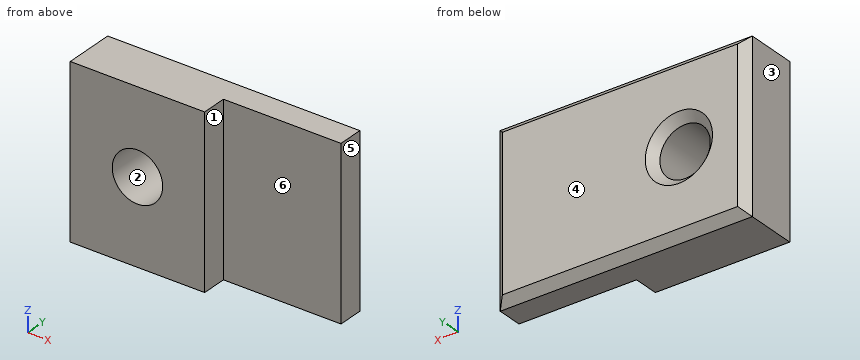
```python
from build123d import *

# Parameters (mm, degrees)
SKETCH1_W           = 30
SKETCH1_H           = 20
SKETCH1_R           = 3
BOSS_EXTRUDE1_DEPTH = 7
SKETCH2_OUTSIDE_W   = 39.346
SKETCH2_OUTSIDE_H   = 29.346
SKETCH2_OUTSIDE_W_2 = 16
SKETCH2_OUTSIDE_H_2 = 20
CUT_EXTRUDE1_DEPTH  = 3
CHAMFER1_SIZE       = 1


with BuildPart() as part:
    # Sketch1 → Boss-Extrude1 (new body)
    with BuildSketch(Plane(origin=(0, 0, 0), x_dir=(1, 0, 0), z_dir=(0, 1, 0))):
        with Locations((7, 0)):
            Rectangle(SKETCH1_W, SKETCH1_H)
        Circle(SKETCH1_R, mode=Mode.SUBTRACT)
    extrude(amount=BOSS_EXTRUDE1_DEPTH)

    # Sketch2 outside → Cut-Extrude1 (cut)
    with BuildSketch(Plane.XZ):
        with Locations((7, 0)):
            Rectangle(SKETCH2_OUTSIDE_W, SKETCH2_OUTSIDE_H)
        Rectangle(SKETCH2_OUTSIDE_W_2, SKETCH2_OUTSIDE_H_2, mode=Mode.SUBTRACT)
    extrude(amount=-CUT_EXTRUDE1_DEPTH, mode=Mode.SUBTRACT)

    # Chamfer1
    chamfer1_edges = [part.edges().sort_by_distance(p)[0] for p in [
        (-3, 7, 0),
        (22, 7, 0),
        (7, 7, -10),
        (-8, 7, 0),
        (7, 7, 10),
    ]]
    chamfer(chamfer1_edges, length=CHAMFER1_SIZE)


solid = part.part
```
Could you check a few things on this model? Use its own coordinates, in mm. Face numbers are marked on the shaded views. A direction names the side the tool comes from. Coordinates: 2 decimals unless noted, no trailing zeros. Loops run counter-clockwise (first coordinate to the right, second up) from the corner with the lowest first, then second, coordinate; pieces in that order, holes last. Notation, with made-up numbers: M -29.75,-8.5 L -20.75,-8.5 A18 ccw -20.75,22.5 Z; hole C 35.5,-16.5 d2. An arc over 180 degrees is marked long. Put each result on its own line as item: value. Start each with the question number.
(1) For the marked faces 5 and 6, which set-ups out of +Z, -Z, +X, -X, +Y, -Y let a thin tool reach every point of the face, with its end or its side?
(2) Will this pin go through, and if not, where does the flat tip stop? P1, Ø0.9, axis at y = 1, z = -3.5, coming from the +X side.
(3) Thinking about a two-plate mould opening in X: for the marked faces 1, 2, 3 and 4, which applies, pulls with the +X half, pulls with the -X half, needs draft (parallel to the pull), parting line crosses it, or undercut?
(4) Suppose I cut it at A-A on z = 0. Please give me the cut outline in (x, y).
(5) Suppose I cut it at B-B on x = 0. Please give me the cut outline in (y, z).
(6) I need wall thicknesses on line 1 (X direction, y = 2.5, z = 0); line 2 (Z direction, x = 0, y = 2.95); line 3 (X direction, y = 3.5, z = 1.25). Which ranges of each line are inside material? Lowest first, please. Write a range as from..to.
(7) Suppose I cut it at C-C on y = 1.75. Please give me the cut outline in (x, z).
(8) Suppose I cut it at D-D on z = -8.5. Please give me the cut outline in (x, y).
Solutions:
1. face 5: +Z, -Z, +X, +Y, -Y
1. face 6: +Z, -Z, +X, -Y
2. P1: stops at x = 8
3. face 1: pulls with the +X half
3. face 2: undercut
3. face 3: pulls with the -X half
3. face 4: needs draft
4. outline: M -8,0 L -3,0 L -3,6 L -4,7 L -7,7 L -8,6 Z; M 3,0 L 8,0 L 8,3 L 22,3 L 22,6 L 21,7 L 4,7 L 3,6 Z
5. outline: M 0,-10 L 6,-10 L 7,-9 L 7,-4 L 6,-3 L 0,-3 Z; M 0,3 L 6,3 L 7,4 L 7,9 L 6,10 L 0,10 Z
6. line 1: x = -8..-3, 3..8
6. line 2: z = -10..-3, 3..10
6. line 3: x = -8..-2.73, 2.73..22
7. outline: M -8,-10 L 8,-10 L 8,10 L -8,10 Z; hole C 0,0 d6
8. outline: M -8,0 L 8,0 L 8,3 L 22,3 L 22,6 L 21,7 L -7,7 L -8,6 Z
